Input: part model. Units: mm. Frame: model coordinates. Face numbers are marked on the shaded views. A direction names the side the tool comes from. Round coordinates to 2 decimals unless told otherwise and drop trailing zeros. Loops run counter-clockwise (first coordinate to the right, second up) from the corner with the lowest first, then second, coordinate; pieces in that order, holes last.
(1) Cut plane C-C, the plane z = 36. Output: boundary loops of the cut face in (x, y).
(2) Cut plane D-D, the plane y = -11. Output: boundary loops of the cut face in (x, z).
(3) Cut plane B-B, the plane x = 22.5. Output: boundary loops of the cut face in (y, z).
(4) Draft query along Z for the marked faces 1, 2 and 3. Return one class per face: released by +Z, released by -Z, zero draft, split by the parting line, or undercut.
(5) Cut plane A-A, the plane y = -17.5. Give the number of separate pieces and of enclosed holes in the cut face, and give its area (3 significant figures).
(6) Access query for the marked faces 4, 5, 6, 7 and 8. Directions: +Z, -Z, +X, -X, +Y, -Y. A direction counts if a zero-diameter tool reaches every point of the face in a straight line with its end or side. Return the directions, or none.
(7) First-contact query: pin 1 Ø3.5 at (x, z) = (14.37, 37.09) entering from -Y; pin 2 Ø1 at (x, z) = (20.5, 16.5) entering from +Y; pin 3 Ø3 at (x, z) = (9, -2) entering from -Y; pin 4 Ø7.5 at (x, z) = (11, 2.5) entering from -Y. Flat tips, straight axial feed; report the tip coordinate or a pass-through.
(8) Line query: line 1 (X direction, y = -17, z = 22.5); line 2 (Z direction, x = 25.5, y = -8.75); line 3 (X direction, y = 5.75, z = 35.5). Output: solid intervals per line, ascending.
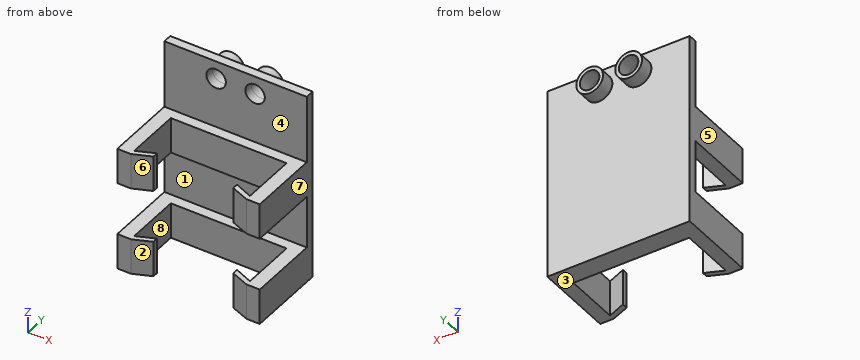
from build123d import *

# Parameters (mm, degrees)
SKETCH3_R           = 2.7813
BOSS_EXTRUDE3_DEPTH = 2.54
SKETCH4_W           = 3.81
SKETCH4_H           = 40.386
BOSS_EXTRUDE4_DEPTH = 20.32
SKETCH5_W           = 40.386
SKETCH5_H           = 1.524
BOSS_EXTRUDE5_DEPTH = 5.08
SKETCH6_W           = 40.386
SKETCH6_H           = 1.524
BOSS_EXTRUDE6_DEPTH = 5.08
SKETCH7_W           = 40.64
SKETCH7_H           = 20.32
CUT_EXTRUDE1_DEPTH  = 5.08
SKETCH11_W          = 40.64
SKETCH11_H          = 35.306
BOSS_EXTRUDE7_DEPTH = 2.9718
BOSS_EXTRUDE8_DEPTH = 35.306
SKETCH8_W           = 14.986
SKETCH8_H           = 20.32
CUT_EXTRUDE2_DEPTH  = 41.64
CUT_EXTRUDE3_DEPTH  = 36.306
SKETCH14_R          = 3.81
SKETCH14_R_2        = 2.7813
BOSS_EXTRUDE9_DEPTH = 6.604


with BuildPart() as part:
    # Sketch3 → Boss-Extrude3 (new body)
    with BuildSketch(Plane(origin=(0, 0, 0), x_dir=(1, 0, 0), z_dir=(0, 1, 0))):
        Polygon((-11.517251908, 12.440983784), (29.122748092, 12.440983784), (29.122748092, -34.564151764), (29.122748092, -42.169016216), (18.885256114, -42.169016216), (-11.517251908, -42.169016216), align=None)
        with Locations((3.240148092, -37.089016216)):
            Circle(SKETCH3_R, mode=Mode.SUBTRACT)
        with Locations((14.365348092, -37.089016216)):
            Circle(SKETCH3_R, mode=Mode.SUBTRACT)
    extrude(amount=BOSS_EXTRUDE3_DEPTH)

    # Sketch4 → Boss-Extrude4 (add)
    with BuildSketch(Plane.XZ):
        with Locations((-9.612251908, 7.752016216)):
            Rectangle(SKETCH4_W, SKETCH4_H)
        with Locations((27.217748092, 7.752016216)):
            Rectangle(SKETCH4_W, SKETCH4_H)
    extrude(amount=BOSS_EXTRUDE4_DEPTH)

    # Sketch5 → Boss-Extrude5 (add)
    with BuildSketch(Plane(origin=(-7.707251908, 0, 0), x_dir=(0, 0, -1), z_dir=(1, 0, 0))):
        with Locations((-7.752016216, -19.558)):
            Rectangle(SKETCH5_W, SKETCH5_H)
    extrude(amount=BOSS_EXTRUDE5_DEPTH)

    # Sketch6 → Boss-Extrude6 (add)
    with BuildSketch(Plane.ZY.offset(-25.312748092)):
        with Locations((7.752016216, -19.558)):
            Rectangle(SKETCH6_W, SKETCH6_H)
    extrude(amount=BOSS_EXTRUDE6_DEPTH)

    # Sketch7 → Cut-Extrude1 (cut)
    with BuildSketch(Plane.XY.offset(27.945016216)):
        with Locations((8.802748092, -10.16)):
            Rectangle(SKETCH7_W, SKETCH7_H)
    extrude(amount=-CUT_EXTRUDE1_DEPTH, mode=Mode.SUBTRACT)

    # Sketch11 → Boss-Extrude7 (add)
    with BuildSketch(Plane.XZ):
        with Locations((8.802748092, 5.212016216)):
            Rectangle(SKETCH11_W, SKETCH11_H)
    extrude(amount=BOSS_EXTRUDE7_DEPTH)

    # Sketch12 → Boss-Extrude8 (add)
    with BuildSketch(Plane.XY.offset(22.865016216)):
        Polygon((-7.707251908, -18.796), (-2.593407451, -16.66881978), (-2.627251908, -18.796), align=None)
        Polygon((20.232748092, -18.796), (20.232748092, -16.66881978), (25.312748092, -18.796), align=None)
    extrude(amount=-BOSS_EXTRUDE8_DEPTH)

    # Sketch8 → Cut-Extrude2 (cut, through all)
    with BuildSketch(Plane(origin=(29.122748092, 0, 0), x_dir=(0, 0, -1), z_dir=(1, 0, 0))):
        with Locations((-5.212016216, -10.16)):
            Rectangle(SKETCH8_W, SKETCH8_H)
    extrude(amount=-CUT_EXTRUDE2_DEPTH, mode=Mode.SUBTRACT)

    # Sketch13 → Cut-Extrude3 (cut, through all)
    with BuildSketch(Plane.XY.offset(22.865016216)):
        Polygon((-2.618031664, -18.216492377), (-7.660745747, -20.32), (-2.627251908, -20.32), (-2.627251908, -18.796), align=None)
        Polygon((20.232748092, -18.294602636), (20.232748092, -20.32), (25.312748092, -20.32), align=None)
    extrude(amount=-CUT_EXTRUDE3_DEPTH, mode=Mode.SUBTRACT)

    # Sketch14 → Boss-Extrude9 (add)
    with BuildSketch(Plane.XZ):
        with Locations((3.240148092, 37.089016216)):
            Circle(SKETCH14_R)
        with Locations((3.240148092, 37.089016216)):
            Circle(SKETCH14_R_2, mode=Mode.SUBTRACT)
        with Locations((14.365348092, 37.089016216)):
            Circle(SKETCH14_R)
        with Locations((14.365348092, 37.089016216)):
            Circle(SKETCH14_R_2, mode=Mode.SUBTRACT)
    extrude(amount=-BOSS_EXTRUDE9_DEPTH)


solid = part.part
Reported:
1. outline: (-11.52, 0) - (0.68, 0) - (0.68, 6.6) - (-0.41, 6.6) - (-0.41, 2.54) - (-11.52, 2.54) - close; (5.8, 0) - (11.81, 0) - (11.81, 6.6) - (10.71, 6.6) - (10.71, 2.54) - (6.89, 2.54) - (6.89, 6.6) - (5.8, 6.6) - close; (16.92, 0) - (29.12, 0) - (29.12, 2.54) - (18.02, 2.54) - (18.02, 6.6) - (16.92, 6.6) - close
2. outline: (-11.52, -12.44) - (-7.71, -12.44) - (-7.71, -2.28) - (-11.52, -2.28) - close; (-11.52, 12.71) - (-7.71, 12.71) - (-7.71, 22.87) - (-11.52, 22.87) - close; (25.31, -12.44) - (29.12, -12.44) - (29.12, -2.28) - (25.31, -2.28) - close; (25.31, 12.71) - (29.12, 12.71) - (29.12, 22.87) - (25.31, 22.87) - close
3. outline: (-19.2, -12.44) - (-17.62, -12.44) - (-17.62, -2.28) - (-19.2, -2.28) - close; (-19.2, 12.71) - (-17.62, 12.71) - (-17.62, 22.87) - (-19.2, 22.87) - close; (-2.97, -12.44) - (2.54, -12.44) - (2.54, 42.17) - (0, 42.17) - (0, 22.87) - (-2.97, 22.87) - (-2.97, 12.71) - (0, 12.71) - (0, -2.28) - (-2.97, -2.28) - close
4. face 1: undercut
4. face 2: zero draft
4. face 3: released by -Z
5. separate pieces: 8
5. enclosed holes: 0
5. area: 236 mm2
6. face 4: +Z, +X, -X, -Y
6. face 5: +Z, -Z, -X, +Y, -Y
6. face 6: +Z, -Z, -Y
6. face 7: +Z, -Z, +X, +Y, -Y
6. face 8: +Z, -Z
7. pin 1: passes through
7. pin 2: stops at y = 2.54
7. pin 3: stops at y = -2.97
7. pin 4: stops at y = 0
8. line 1: x = -11.52 to -7.71, -3.39 to -2.6, 20.23 to 21.02, 25.31 to 29.12
8. line 2: z = -12.44 to -2.28, 12.71 to 22.87
8. line 3: x = -0.22 to 0.96, 5.52 to 6.7, 10.9 to 12.08, 16.65 to 17.83
